from build123d import *

# Parameters (mm, degrees)
F0_R     = 25
F1_DEPTH = 18
F2_R     = 12
F3_DEPTH = 2
F4_R     = 8
F5_DEPTH = 25
F6_R     = 2.5


with BuildPart() as f1:
    # F0 (on Top) → F1 (new body)
    with BuildSketch(Plane.XY):
        Circle(F0_R)
    extrude(amount=F1_DEPTH)

    # F2 (on face) → F3 (join)
    with BuildSketch(Plane.XY.offset(18)):
        Circle(F2_R)
    extrude(amount=F3_DEPTH)

    # F4 (on face) → F5 (cut)
    with BuildSketch(Plane.XY.offset(20)):
        Circle(F4_R)
    extrude(amount=-F5_DEPTH, mode=Mode.SUBTRACT)

    # F6 (on Front) → F8 (revolve, cut)
    with BuildSketch(Plane.XZ):
        with Locations((25, 13)):
            Circle(F6_R)
        with Locations((25, 5)):
            Circle(F6_R)
    revolve(axis=Axis((0, 0, 7.756283), (0, 0, -1)), mode=Mode.SUBTRACT)


solid = f1.part
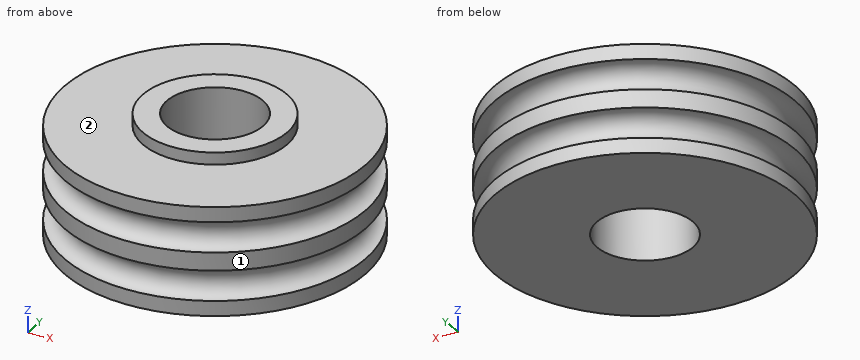
CAD build for the part. Positions are in the model's coordinates, mm. Face numbers are marked on the shaded views. A direction names the side the tool comes from. Round coordinates to 2 decimals unless told otherwise and drop trailing zeros. Order: outer loops, then holes, each group sorted by start corner. A loop starts at its lowest first (then second) coordinate and runs counter-clockwise, first axis right, second up. Notation, with made-up numbers: (-33, -24) - (-26, -24) arc R6 ccw to (-26, -19) - close; hole circle Ø9 at (27.5, -10.5). An arc over 180 degrees is marked (long way). Return JSON: item names as keys, results as strings.
(1) Cut at A-A (y = 0). Give the cut face in (x, z).
Answer key:
{"outline": "(-25, 0) - (-8, 0) - (-8, 20) - (-12, 20) - (-12, 18) - (-25, 18) - (-25, 15.5) arc R2.5 cw to (-25, 10.5) - (-25, 7.5) arc R2.5 cw to (-25, 2.5) - close; (8, 0) - (25, 0) - (25, 2.5) arc R2.5 cw to (25, 7.5) - (25, 10.5) arc R2.5 cw to (25, 15.5) - (25, 18) - (12, 18) - (12, 20) - (8, 20) - close"}
(2) Cut at C-C (z = 9). Give the cut face in (x, y).
Answer key:
{"outline": "circle Ø50 at (0, 0); hole circle Ø16 at (0, 0)"}
(3) Wall check: probe 1 along Z at (x, y) = (-13, -21); probe 2 along Z at (x, y) = (13.5, 0); probe 3 along Z at (x, y) = (-23, 5). Give the ranges that are in metal, low to high. Write a range as from..to.
Answer key:
{"probe 1": "z = 0..2.52, 7.48..10.52, 15.48..18", "probe 2": "z = 0..18", "probe 3": "z = 0..2.97, 7.03..10.97, 15.03..18"}
(4) Tool access for the marked faces 1 and 2: list every direction of +Z, -Z, +X, -X, +Y, -Y with a clear straight run to the whole face (end or side of a thin tool).
Answer key:
{"face 1": "+Z, -Z", "face 2": "+Z"}
(5) Cut at D-D (z = 3.5). Give the cut face in (x, y).
Answer key:
{"outline": "circle Ø46 at (0, 0); hole circle Ø16 at (0, 0)"}
(6) Pin check, flat tips, straight feed: pin 1 Ø3 at (x, y) = (10, -17.5) entering from +Z; pin 2 Ø12 at (y, z) = (-9.5, 13) entering from +X; pin 3 Ø1.5 at (y, z) = (-12, 16.5) entering from +X; pin 4 Ø9.5 at (x, y) = (0, 0) entering from -Z. Stop position of each tip, or through.
Answer key:
{"pin 1": "stops at z = 18", "pin 2": "stops at x = 24.67", "pin 3": "stops at x = 22.33", "pin 4": "passes through"}
